The model under review builds one solid part; all positions refer to its coordinate system, in mm. A direction names the side the tool comes from. Coordinates: 2 decimals unless noted, no trailing zeros. Loops run counter-clockwise (first coordinate to the right, second up) from the corner with the lowest first, then second, coordinate; pieces in that order, holes last. Notation, with made-up numbers: (40, -24) - (93, -24) arc R29 ccw to (93, 11) - close; hole circle Ø8 at (-4, 57). An arc over 180 degrees is marked (long way). One line per item, written item: value. Start each with the question number.
1. We need section A-A, the plane x = 0. Give the boundary of the cut face in (y, z), then the cut area to 3 significant figures.
2. For faces 5 (the face through (5.5, -2.5, 11.2)), 6 (the face through (3, 0, 10)), 7 (the face through (-5.5, -2.5, 10.8)), 8 (the face through (0, 1, 4)), 9 (the face through (0, 0, 15)), list the 3-axis set-ups (+Z, -Z, +X, -X, +Y, -Y) from which the entire face can be reached by the end or side of a thin tool; tool diameter is ignored.
3. We need section B-B, the plane y = -0.5. Give the boundary of the cut face in (x, z).
4. Insertion check: P1, Ø4, axis at x = 2.5, y = 2, coming from the +Z side; P2, Ø3.5, axis at y = -1, z = 10, coming from the +X side; P3, Ø1.5, axis at y = -0.5, z = 12, coming from the -X side. Each pin has a flat end and moves straight along its axis. Give the tip position at first contact, or say it passes through.
5. To check wall thickness, follow line 1 (Z direction, x = 0, y = 0.75); line 2 (Z direction, x = 0, y = 1.25). State the ranges of each line that lie inside material, in increasing order.
6. Mouldability with a two-part tool opening along X and no side actions: class faces 1 (the face through (-4.787, -2.493, 16.748)), 2 (the face through (5.682, -2.493, 6.614)), 3 (the face through (0, -2.5, 17.5)), 4 (the face through (-1.9, 0.55, -0.08)) as +X half, -X half, draft (parallel to the pull), parting line (faces both ways), or undercut.
7. We need section C-C, the plane z = 12.25. Give the boundary of the cut face in (x, y), then the cut area to 3 significant figures.
8. We need section D-D, the plane z = -0.75. Give the boundary of the cut face in (x, y), then the cut area to 3 significant figures.
Autodesk Inventor part; units mm, degrees
ref_plane "YZ Plane" through (0, 0, 0) normal (1, 0, 0) x (0, 1, 0)
ref_plane "XZ Plane" through (0, 0, 0) normal (0, 1, 0) x (-1, 0, 0)
ref_plane "XY Plane" through (0, 0, 0) normal (0, 0, 1) x (1, 0, 0)
sketch "スケッチ1" plane through (0, 0, 0) normal (0, 1, 0) x (-1, 0, 0)
  circle A0 centre (0, 0) radius 6
  dimension "d0" = 12
extrude "押し出し1" add sketch "スケッチ1" along normal blind 1
sketch "スケッチ2" plane through (0, 1, 0) normal (0, 1, 0) x (1, 0, 0)
  circle A0 centre (0, 0) radius 3
  dimension "d3" = 6
extrude "押し出し2" add sketch "スケッチ2" along normal blind 3
sketch "スケッチ3" plane through (0, 4, 0) normal (0, 1, 0) x (1, 0, 0)
  circle A0 centre (0, 0) radius 1.9
  dimension "d6" = 3.8
extrude "押し出し3" cut sketch "スケッチ3" against normal through all
sketch "スケッチ5" plane through (0, 1, 0) normal (0, 1, 0) x (1, 0, 0)
  circle A0 centre (0, 0) radius 3
  circle A1 centre (0, 0) radius 6
  line L0 (-3, 0) -> (3, 0)
  line L1 (3, 0) -> (3, -15)
  line L2 (3, -15) -> (-3, -15)
  line L3 (-3, -15) -> (-3, 0)
  circle A2 centre (0, 0) radius 3
  circle A3 centre (0, 0) radius 1.9
  point P0 (3, -5.1962)
  point P1 (-3, -5.1962)
  dimension "d9" = 15
extrude "押し出し4" add sketch "スケッチ5" against normal blind 3 contours L0 A3 A0 | L1 A1 L3 A0 | A0 L0 A3 | A0 L3 A1 L1 | L1 L2 L3 A1
sketch "スケッチ6" plane through (0, -2, 0) normal (0, -1, 0) x (1, 0, 0)
  line L0 (5.5, 17.5) -> (-5.5, 17.5)
  line L1 (-5.5, 17.5) -> (-5.5, 0)
  line L2 (-5.5, 0) -> (5.5, 0)
  line L3 (5.5, 0) -> (5.5, 17.5)
  line L4 (3, 5.1962) -> (3, 15)
  line L5 (-3, 15) -> (-3, 5.1962)
  line L6 (3, 15) -> (-3, 15)
  arc A0 (-3, 5.1962) -> (3, 5.1962) centre (0, 0) ccw
  circle A1 centre (0, 0) radius 8.5
  circle A2 centre (0, 0) radius 1.9
  line L7 (-6, -6.0208) -> (-6, 6.0208)
  point P0 (-5.5, 6.4807)
  point P1 (5.5, 6.4807)
  dimension "d12" = 2.5
  dimension "d13" = 2.5
  dimension "d14" = 2.5
  dimension "d15" = 2.5
extrude "押し出し5" add sketch "スケッチ6" along normal blind 1 contours L3 A1 L4 L6 L5 L1 L0 | A1 L7 A0 L3 | L3 A0 L4 A1 | A1 L5 A0 L1 | L1 A0 L7 A1 | A0 L1 L2 A2 L3 | L3 L2 A2 L1 A0 L5 A1 L4 | A1 L5 L6 L4
fillet "フィレット1" radius 2.5 5 edges at (5.5, -2.5, 17.5) (-5.5, -2.5, 17.5) (-6, -2.5, 6.0208) (-6, -2.5, -6.0208) (5.5, -2.5, 6.4807)
properties part number "ベルト_bush_皿側"
Findings below:
1. outline: (-3, -8.5) - (-2, -8.5) - (-2, -6) - (1, -6) - (1, -3) - (4, -3) - (4, -1.9) - (-3, -1.9) - close; (-3, 1.9) - (4, 1.9) - (4, 3) - (1, 3) - (1, 15) - (-2, 15) - (-2, 17.5) - (-3, 17.5) - close
1. area: 80.4 mm2
2. face 5: +Z, +X, +Y, -Y
2. face 6: +Z, +X, +Y
2. face 7: +Z, -X, +Y, -Y
2. face 8: +Y
2. face 9: +Z, +X, -X, +Y
3. outline: (-3, 5.2) arc R6 ccw (long way) to (3, 5.2) - (3, 15) - (-3, 15) - close; hole circle Ø3.8 at (0, 0)
4. P1: z = 15
4. P2: x = 5.5
4. P3: x = -3
5. line 1: -6 to -1.9, 1.9 to 15
5. line 2: -3 to -1.9, 1.9 to 3
6. face 1: -X half
6. face 2: +X half
6. face 3: draft
6. face 4: undercut
7. outline: (-5.5, -3) - (5.5, -3) - (5.5, -2) - (3, -2) - (3, 1) - (-3, 1) - (-3, -2) - (-5.5, -2) - close
7. area: 29.0 mm2
8. outline: (-6, -3) - (-1.75, -3) - (-1.75, 4) - (-2.9, 4) - (-2.9, 1) - (-5.95, 1) - (-5.95, -2) - (-6, -2) - close; (1.75, -3) - (8.47, -3) - (8.47, -2) - (5.95, -2) - (5.95, 1) - (2.9, 1) - (2.9, 4) - (1.75, 4) - close
8. area: 43.2 mm2
